For this review, take the finished solid that the model builds, in its own axes (mm). A direction names the side the tool comes from. Give positions to 0.01 mm unless a question says otherwise; leave off trailing zeros. Order: outer loops, then holes, each group sorted by start corner. A loop starts at its lowest first (then second) coordinate and runs counter-clockwise, first axis right, second up. Notation, with made-up numbers: M -5.5,2 L 45.5,2 A26 cw 45.5,26 Z; hole C 67,29.5 d9. An arc over 180 degrees is marked long. Use CSV: the item, a comma, the result in double quotes. Start each with the question number.
(1) Consider section D-D (z = 47.5). Write out the cut boundary in (x, y).
(2) Consider section A-A (z = 8.5). Write out the cut boundary in (x, y), and give its area (3 significant figures).
(3) Clearance check with flat-ended pins moving along their axes: P1, Ø15, axis at y = -25.5, z = 25, coming from the -X side; P2, Ø12, axis at y = -10.5, z = 40, coming from the +X side; P3, Ø20.5, axis at x = 63.5, y = -9, coming from the +Z side. State where each tip first meets the part, or that it passes through.
(4) Tool access review of faces 1 (the face through (58, -69, 12.7)), 2 (the face through (-63.1, -12.26, 6.44)), 3 (the face through (63.897, -13.196, 6.439)): name each direction out of +Z, -Z, +X, -X, +Y, -Y from which nothing blocks a thin tool from reaching the whole face with its end or side.
(5) Wall thickness on L1, parallel to X at y = -71, z = 14; L2, parallel to X at y = -13, z = 39.5; L3, parallel to Y at x = -49, z = 36.5: over which ranges is each line inside the solid? List them lowest first. Write a range as from..to.
(6) Consider section B-B (x = 44). Write out the cut boundary in (y, z), and give its area (3 significant figures).
(7) Consider section C-C (y = -20). Write out the cut boundary in (x, z).
(8) Draft analysis for pull direction Y (two halves, no side actions). For faces 4 (the face through (-1, 0, 31)), 5 (the face through (38.319, -38, 10)), 6 (the face through (0.93, -47.754, 42.498)), state which applies: pulls with the +Y half, pulls with the -Y half, needs draft (parallel to the pull), parting line crosses it, or undercut.
```python
from build123d import *

# Parameters (mm, degrees)
F1_DEPTH = 76.2
F3_DEPTH = 12.7
F5_DEPTH = 12.7
F7_DEPTH = 101.6


with BuildPart() as f1:
    # F0 (on Front) → F1 (new body)
    with BuildSketch(Plane.XZ):
        Polygon((-75.980723, 12.7), (-75.980723, 0), (-37.880723, 0), (-37.880723, 19.05), (38.319277, 19.05), (38.319277, 0), (76.419277, 0), (76.419277, 12.7), (51.019277, 12.7), (51.019277, 50.8), (-50.580723, 50.8), (-50.580723, 12.7), align=None)
    extrude(amount=F1_DEPTH)

    # F2 (on face) → F3 (cut, through all)
    with BuildSketch(Plane.XY.offset(12.7)):
        Polygon((51.019277, -50.941616), (76.419277, -76.2), (76.419277, 0), (51.019277, -26.765935), align=None)
    extrude(amount=-F3_DEPTH, mode=Mode.SUBTRACT)

    # F4 (on face) → F5 (cut, through all)
    with BuildSketch(Plane.XY.offset(12.7)):
        Polygon((-75.980723, 0), (-75.980723, -76.2), (-50.580723, -51.805038), (-50.580723, -24.175685), align=None)
    extrude(amount=-F5_DEPTH, mode=Mode.SUBTRACT)

    # F6 (on face) → F7 (cut, through all)
    with BuildSketch(Plane.YZ.offset(51.019277)):
        Polygon((-56.127969, 50.8), (-39.141584, 33.96108), (-22.448849, 50.8), align=None)
    extrude(amount=-F7_DEPTH, mode=Mode.SUBTRACT)


solid = f1.part
```
Check result:
1,outline,"M -50.58,-76.2 L 51.02,-76.2 L 51.02,-52.8 L -50.58,-52.8 Z; M -50.58,-25.72 L 51.02,-25.72 L 51.02,0 L -50.58,0 Z"
2,outline,"M -75.98,-76.2 L -37.88,-76.2 L -37.88,0 L -75.98,0 L -50.58,-24.18 L -50.58,-51.81 Z; M 38.32,-76.2 L 76.42,-76.2 L 51.02,-50.94 L 51.02,-26.77 L 76.42,0 L 38.32,0 Z"
2,area,"3,210 mm^2"
3,P1,"stops at x = -50.58"
3,P2,"stops at x = 51.02"
3,P3,"stops at z = 12.7"
4,face 1,"+Z, +X, +Y, -Y"
4,face 2,"+Z, -Z, -X"
4,face 3,"+Z, -Z, +X"
5,L1,"x = -50.58..-37.88, 38.32..51.02"
5,L2,"x = -50.58..51.02"
5,L3,"y = -76.2..-41.7, -36.62..0"
6,outline,"M -76.2,0 L 0,0 L 0,50.8 L -22.45,50.8 L -39.14,33.96 L -56.13,50.8 L -76.2,50.8 Z"
6,area,"3,590 mm^2"
7,outline,"M -54.97,0 L -37.88,0 L -37.88,19.05 L 38.32,19.05 L 38.32,0 L 57.44,0 L 57.44,12.7 L 51.02,12.7 L 51.02,50.8 L -50.58,50.8 L -50.58,12.7 L -54.97,12.7 Z"
8,face 4,"pulls with the +Y half"
8,face 5,"needs draft"
8,face 6,"undercut"
